Check sheet for the modelled part. Datum: model origin and axes. Units: mm. Round coordinates to 2 decimals unless told otherwise and drop trailing zeros. Put each result on its own line as item: value.
```python
from build123d import *

# Parameters (mm, degrees)
F0_W     = 45
F0_H     = 0.01
F0_W_2   = 0.01
F0_H_2   = 35
F1_DEPTH = 6
F1_TAPER = -15


with BuildPart() as f1:
    # F0 (on Top) → F1 (new body)
    with BuildSketch(Plane.XY):
        with Locations((67.51, 105.025)):
            Rectangle(F0_W, F0_H)
        Polygon((90.02, 0), (90.02, -0.01), (135.03, -0.01), (135.03, 35), (135.02, 35), (135.02, 0), align=None)
        Polygon((-0.01, 105.03), (-0.01, 70.02), (0, 70.02), (0, 105.02), (45, 105.02), (45, 105.03), align=None)
        with Locations((-0.005, 52.51)):
            Rectangle(F0_W_2, F0_H_2)
        Polygon((45, 0), (0, 0), (0, 35), (-0.01, 35), (-0.01, -0.01), (45, -0.01), align=None)
        Polygon((90.02, 105.03), (90.02, 105.02), (135.02, 105.02), (135.02, 70.02), (135.03, 70.02), (135.03, 105.03), align=None)
        with Locations((135.025, 52.51)):
            Rectangle(F0_W_2, F0_H_2)
        with Locations((67.51, -0.005)):
            Rectangle(F0_W, F0_H)
        Polygon((-0.01, 35), (0, 35), (45, 35), (45, 35.01), (0, 35.01), (-0.01, 35.01), align=None)
        with Locations((90.015, 52.51)):
            Rectangle(F0_W_2, F0_H_2)
        Polygon((90.02, 35), (90.01, 35), (90.01, 0), (90.01, -0.01), (90.02, -0.01), (90.02, 0), align=None)
        Polygon((45, 105.02), (45, 70.02), (45.01, 70.02), (45.01, 105.02), (45.01, 105.03), (45, 105.03), align=None)
        Polygon((45, 35), (45, 0), (45, -0.01), (45.01, -0.01), (45.01, 0), (45.01, 35), align=None)
        Polygon((90.01, 105.02), (90.01, 70.02), (90.02, 70.02), (90.02, 105.02), (90.02, 105.03), (90.01, 105.03), align=None)
        with Locations((67.51, 70.015)):
            Rectangle(F0_W, F0_H)
        with Locations((45.005, 52.51)):
            Rectangle(F0_W_2, F0_H_2)
        with Locations((67.51, 35.005)):
            Rectangle(F0_W, F0_H)
        Polygon((90.02, 70.02), (90.02, 70.01), (135.02, 70.01), (135.03, 70.01), (135.03, 70.02), (135.02, 70.02), align=None)
        Polygon((90.02, 35.01), (90.02, 35), (135.02, 35), (135.03, 35), (135.03, 35.01), (135.02, 35.01), align=None)
        Polygon((0, 70.01), (45, 70.01), (45, 70.02), (0, 70.02), (-0.01, 70.02), (-0.01, 70.01), align=None)
        with Locations((90.015, 35.005)):
            Rectangle(F0_W_2, F0_H)
        with Locations((45.005, 70.015)):
            Rectangle(F0_W_2, F0_H)
        with Locations((45.005, 35.005)):
            Rectangle(F0_W_2, F0_H)
        with Locations((90.015, 70.015)):
            Rectangle(F0_W_2, F0_H)
    extrude(amount=F1_DEPTH, taper=F1_TAPER)


solid = f1.part
```
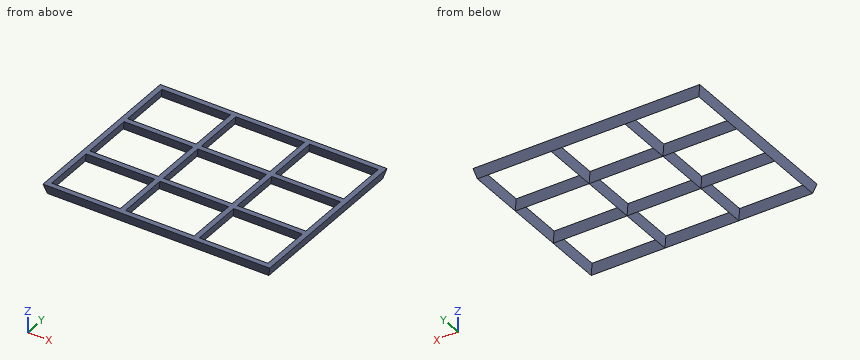
Item 1: Section check A-A on x = 54.5. Count the separate pieces of the cut face and the enclosed holes in it, then the cut area to 3 significant figures.
Filled sheet:
separate pieces: 4
enclosed holes: 0
area: 38.8 mm²
Item 2: Go/stop test with flat-tipped pins: pin 1 (12 mm diameter, centred on x = 121.5, y = 25, fed in from -Z); pin 2 (8 mm diameter, centred on x = 102, y = 64.5, fed in from +Z). Record where each tip stops, or that it passes through.
Filled sheet:
pin 1: through
pin 2: z = 6
Item 3: Thickness scan on line 1 (X direction, y = 76, z = 5.75); line 2 (Y direction, x = 73.5, z = 3); line 3 (Y direction, x = 100, z = 3.5). Record the ranges inside material, lowest first. Write a range as from..to.
Filled sheet:
line 1: -1.55..1.54, 43.46..46.55, 88.47..91.56, 133.48..136.57
line 2: -0.81..0.8, 34.2..35.81, 69.21..70.82, 104.22..105.83
line 3: -0.95..0.94, 34.06..35.95, 69.07..70.96, 104.08..105.97
